Build history of the part. All positions in model axes, mm. A direction names the side the tool comes from. Coordinates: 2 decimals unless noted, no trailing zeros. Loops run counter-clockwise (first coordinate to the right, second up) from the corner with the lowest first, then second, coordinate; pieces in that order, holes last.
(1) Tool access for faces 5 (the face through (31, -20.014, 3)), 6 (the face through (21.978, -17.514, 2.535)): list every direction of +Z, -Z, +X, -X, +Y, -Y with a clear straight run to the whole face (end or side of a thin tool).
(2) Wall check: L1, parallel to Y at x = -24, z = 2.25; L2, parallel to Y at x = 24, z = 3.05; L3, parallel to Y at x = 3.5, z = 0.9. Give the ranges that are in metal, low to high.
(3) Slice it at A-A (x = 0). Give the cut face in (y, z).
(4) Slice it at B-B (y = -6). Give the cut face in (x, z).
(5) Flat gauge pins, fed straight in: P1, Ø4, axis at x = -10.92, y = -12.99, coming from the -Z side; P2, Ø3, axis at y = -6.5, z = 3.5, coming from the +X side; P3, Ø3, axis at x = -17.5, z = 2, coming from the +Y side; P4, Ø0.9, axis at y = -21, z = 2, coming from the +X side. Where does each tip first touch, or does it go through?
(6) Two-plate mould, pull along X, no slides. Class faces 1 (the face through (-0.195, 18.558, 2.465)), 2 (the face through (29, -24, 3)), 3 (the face through (-24, -20.014, 3)), 4 (the face through (32.396, -15, 2)): pulls with the +X half, pulls with the -X half, needs draft (parallel to the pull), parting line crosses it, or undercut.
(7) Slice it at D-D (y = 6.5). Give the cut face in (x, z), and give its area (3 significant figures).
from build123d import *

# Parameters (mm, degrees)
SKETCH1_R           = 3.5
SKETCH1_R_2         = 1.5
BOSS_EXTRUDE1_DEPTH = 5
SKETCH2_W           = 3
SKETCH2_H           = 8
SKETCH2_W_2         = 16
SKETCH2_H_2         = 3
CUT_EXTRUDE3_DEPTH  = 10
SKETCH4_OUTSIDE_W   = 83.878
SKETCH4_OUTSIDE_H   = 74.539
CUT_EXTRUDE5_DEPTH  = 10
BOSS_EXTRUDE2_DEPTH = 5
SKETCH5_R           = 1
CUT_EXTRUDE6_DEPTH  = 5
CUT_EXTRUDE7_DEPTH  = 6


with BuildPart() as part:
    # Sketch1 → Boss-Extrude1 (new body)
    with BuildSketch(Plane.XY):
        with BuildLine():
            Line((16.678684739, -6.865443356), (7.048954955, 19.63254949))
            ThreePointArc((7.048954955, 19.63254949), (-0.000574134, 24.570863688), (-7.049347073, 19.631470247))
            Line((-7.049347073, 19.631470247), (-16.60248251, -6.668301445))
            ThreePointArc((-16.60248251, -6.668301445), (-23.589225287, -5.352701736), (-28.111762071, -10.838322782))
            Line((-28.111762071, -10.838322782), (-32.396038203, -10.838322782))
            Line((-32.396038203, -10.838322782), (-32.396038203, -30.881690835))
            Line((-32.396038203, -30.881690835), (32.396038203, -30.881690835))
            Line((32.396038203, -30.881690835), (32.396038203, -10.838322782))
            Line((32.396038203, -10.838322782), (28.403544795, -10.838322782))
            ThreePointArc((28.403544795, -10.838322782), (23.74315896, -5.304380506), (16.678684739, -6.865443356))
        make_face()
        with BuildLine():
            Line((18.109177542, -10.838322782), (18.172818569, -10.838322782))
            ThreePointArc((18.172818569, -10.838322782), (24.845541744, -12.952957548), (18.140100673, -10.944481806))
            ThreePointArc((18.140100673, -10.944481806), (18.124834746, -10.891345307), (18.109177542, -10.838322782))
        make_face(mode=Mode.SUBTRACT)
        with BuildLine():
            ThreePointArc((-10.753093745, -20.488849886), (-10.919568848, -20.490697711), (-11.086043951, -20.488849886))
            Line((-11.086043951, -20.488849886), (-10.753093745, -20.488849886))
        make_face(mode=Mode.SUBTRACT)
        with Locations((-21.209007359, -11.922115015)):
            Circle(SKETCH1_R, mode=Mode.SUBTRACT)
        with BuildLine():
            Line((3.592595297, 8.251863973), (8.245757774, 8.254276772))
            Line((8.245757774, 8.254276772), (8.248133809, 3.67201473))
            ThreePointArc((8.248133809, 3.67201473), (8.625435504, 2.640272663), (8.874223719, 1.570248043))
            ThreePointArc((8.874223719, 1.570248043), (10.249998622, 0.076178628), (8.875773895, -1.41931674))
            ThreePointArc((8.875773895, -1.41931674), (8.62809549, -2.489598792), (8.251863973, -3.521731588))
            Line((8.251863973, -3.521731588), (8.254313497, -8.24572101))
            Line((8.254313497, -8.24572101), (3.601151021, -8.248133809))
            ThreePointArc((3.601151021, -8.248133809), (0.004666758, -8.99999879), (-3.592595297, -8.251863973))
            Line((-3.592595297, -8.251863973), (-8.245721029, -8.254276752))
            Line((-8.245721029, -8.254276752), (-8.248133809, -3.601151021))
            ThreePointArc((-8.248133809, -3.601151021), (-8.625435504, -2.569408953), (-8.874223719, -1.499384334))
            ThreePointArc((-8.874223719, -1.499384334), (-10.249998622, -0.005314919), (-8.875773895, 1.49018045))
            ThreePointArc((-8.875773895, 1.49018045), (-8.62809549, 2.560462502), (-8.251863973, 3.592595297))
            Line((-8.251863973, 3.592595297), (-8.254276752, 8.245721029))
            Line((-8.254276752, 8.245721029), (-3.601151021, 8.248133809))
            ThreePointArc((-3.601151021, 8.248133809), (-0.004666758, 8.99999879), (3.592595297, 8.251863973))
        make_face(mode=Mode.SUBTRACT)
        with Locations((0, 17.070863709)):
            Circle(SKETCH1_R_2, mode=Mode.SUBTRACT)
        with Locations((-10.919568848, -12.990697711)):
            Circle(SKETCH1_R_2, mode=Mode.SUBTRACT)
        with Locations((10.924107384, -12.988849886)):
            Circle(SKETCH1_R_2, mode=Mode.SUBTRACT)
    extrude(amount=BOSS_EXTRUDE1_DEPTH)

    # Sketch2 → Cut-Extrude3 (cut)
    with BuildSketch(Plane.XY.offset(5)):
        with Locations((27.500296009, -21.513780425)):
            Rectangle(SKETCH2_W, SKETCH2_H)
        with Locations((24.396038203, -21.513780425)):
            Rectangle(SKETCH2_W_2, SKETCH2_H_2)
        with BuildLine():
            Line((23.000296009, -18.513780425), (23.000296009, -24.513780425))
            ThreePointArc((23.000296009, -24.513780425), (22.000296009, -25.513780425), (21.000296009, -24.513780425))
            Line((21.000296009, -24.513780425), (21.000296009, -18.513780425))
            ThreePointArc((21.000296009, -18.513780425), (22.000296009, -17.513780425), (23.000296009, -18.513780425))
        make_face()
    cut_extrude3 = extrude(amount=-CUT_EXTRUDE3_DEPTH, mode=Mode.SUBTRACT)

    # Mirror1: Cut-Extrude3 across plane
    add(cut_extrude3.mirror(Plane(origin=(0, 0, 0), x_dir=(0, 0, 1), z_dir=(1, 0, 0))), mode=Mode.SUBTRACT)

    # Sketch4 outside → Cut-Extrude5 (cut)
    with BuildSketch(Plane.XY.offset(5)):
        with Locations((0, -3.1555)):
            Rectangle(SKETCH4_OUTSIDE_W, SKETCH4_OUTSIDE_H)
        with BuildLine():
            Line((-32.396038203, -10.838322782), (-17.497591027, 11.611817612))
            ThreePointArc((-17.497591027, 11.611817612), (0, 21), (17.497591027, 11.611817612))
            Line((17.497591027, 11.611817612), (32.396038203, -10.838322782))
            Line((32.396038203, -10.838322782), (32.396038203, -30.881690835))
            Line((32.396038203, -30.881690835), (-32.396038203, -30.881690835))
            Line((-32.396038203, -30.881690835), (-32.396038203, -10.838322782))
        make_face(mode=Mode.SUBTRACT)
    extrude(amount=-CUT_EXTRUDE5_DEPTH, mode=Mode.SUBTRACT)

    # Sketch4_5 → Boss-Extrude2 (add)
    with BuildSketch(Plane.XY.offset(5)):
        with BuildLine():
            Line((-17.497591027, 11.611817612), (-32.396038203, -10.838322782))
            Line((-32.396038203, -10.838322782), (-28.111762071, -10.838322782))
            ThreePointArc((-28.111762071, -10.838322782), (-23.589225287, -5.352701736), (-16.60248251, -6.668301445))
            Line((-16.60248251, -6.668301445), (-7.049347073, 19.631470247))
            Line((-7.049347073, 19.631470247), (-6.984017788, 19.804633184))
            ThreePointArc((-6.984017788, 19.804633184), (-12.90805366, 16.564484619), (-17.497591027, 11.611817612))
        make_face()
        with BuildLine():
            ThreePointArc((17.497591027, 11.611817612), (12.90805366, 16.564484619), (6.984017788, 19.804633184))
            Line((6.984017788, 19.804633184), (7.048954955, 19.63254949))
            Line((7.048954955, 19.63254949), (16.678684739, -6.865443356))
            ThreePointArc((16.678684739, -6.865443356), (23.74315896, -5.304380506), (28.403544795, -10.838322782))
            Line((28.403544795, -10.838322782), (32.396038203, -10.838322782))
            Line((32.396038203, -10.838322782), (17.497591027, 11.611817612))
        make_face()
    extrude(amount=-BOSS_EXTRUDE2_DEPTH)

    # Sketch5 → Cut-Extrude6 (cut)
    with BuildSketch(Plane.XY.offset(5)):
        with Locations((0.014555548, -27.999996217)):
            Circle(SKETCH5_R)
        with Locations((20.014552859, -27.989625643)):
            Circle(SKETCH5_R)
        with Locations((-19.985441764, -28.01036679)):
            Circle(SKETCH5_R)
    extrude(amount=-CUT_EXTRUDE6_DEPTH, mode=Mode.SUBTRACT)

    # Sketch6 → Cut-Extrude7 (cut, through all)
    with BuildSketch(Plane.XY.offset(5)):
        with BuildLine():
            ThreePointArc((-32.396038203, -10.838322782), (-21.107946915, -2.160816504), (-17.497591027, 11.611817612))
            ThreePointArc((-17.497591027, 11.611817612), (-30.842179781, 4.299051969), (-32.396038203, -10.838322782))
        make_face()
        with BuildLine():
            ThreePointArc((32.396038203, -10.838322782), (21.107946915, -2.160816504), (17.497591027, 11.611817612))
            ThreePointArc((17.497591027, 11.611817612), (30.860111099, 4.310951618), (32.396038203, -10.838322782))
        make_face()
    extrude(amount=-CUT_EXTRUDE7_DEPTH, mode=Mode.SUBTRACT)


solid = part.part
Response values:
1. face 5: +Z, -Z, +X
1. face 6: +Z, -Z
2. L1: y = -30.88 to -23.01, -20.01 to -14.03, -9.81 to -5.67
2. L2: y = -30.88 to -23.01, -20.01 to -14.37, -9.47 to -5.67
2. L3: y = -30.88 to -8.29, 8.29 to 20.71
3. outline: (-30.88, 0) - (-29, 0) - (-29, 5) - (-30.88, 5) - close; (-27, 0) - (-9, 0) - (-9, 5) - (-27, 5) - close; (9, 0) - (15.57, 0) - (15.57, 5) - (9, 5) - close; (18.57, 0) - (21, 0) - (21, 5) - (18.57, 5) - close
4. outline: (-24.34, 0) - (-8.25, 0) - (-8.25, 5) - (-24.34, 5) - close; (8.25, 0) - (24.34, 0) - (24.34, 5) - (8.25, 5) - close
5. P1: stops at z = 0
5. P2: stops at x = 26.8
5. P3: stops at y = 13.6
5. P4: stops at x = 16.4
6. face 1: undercut
6. face 2: undercut
6. face 3: needs draft
6. face 4: pulls with the +X half
7. outline: (-17.72, 0) - (-8.25, 0) - (-8.25, 5) - (-17.72, 5) - close; (8.25, 0) - (17.72, 0) - (17.72, 5) - (8.25, 5) - close
7. area: 94.7 mm2
